Source: three-view drawing plus pictorial views. Frame: mm from the lowest corner of the part. A direction names the side the tool comes from. Give positions to 0.01 mm unless a question says otherwise; leave off trailing zeros. Loops run counter-clockwise (first coordinate to the right, second up) from the corner with the lowest first, then second, coordinate; pieces in that order, holes last. Notation, with made-up numbers: (80, 34) - (105, 34) arc R24 cw to (105, 49) - close; hole circle Ø1 at (7.5, 84.25). An arc over 180 degrees is marked (long way). Answer as a JSON object with one key per item and string values.
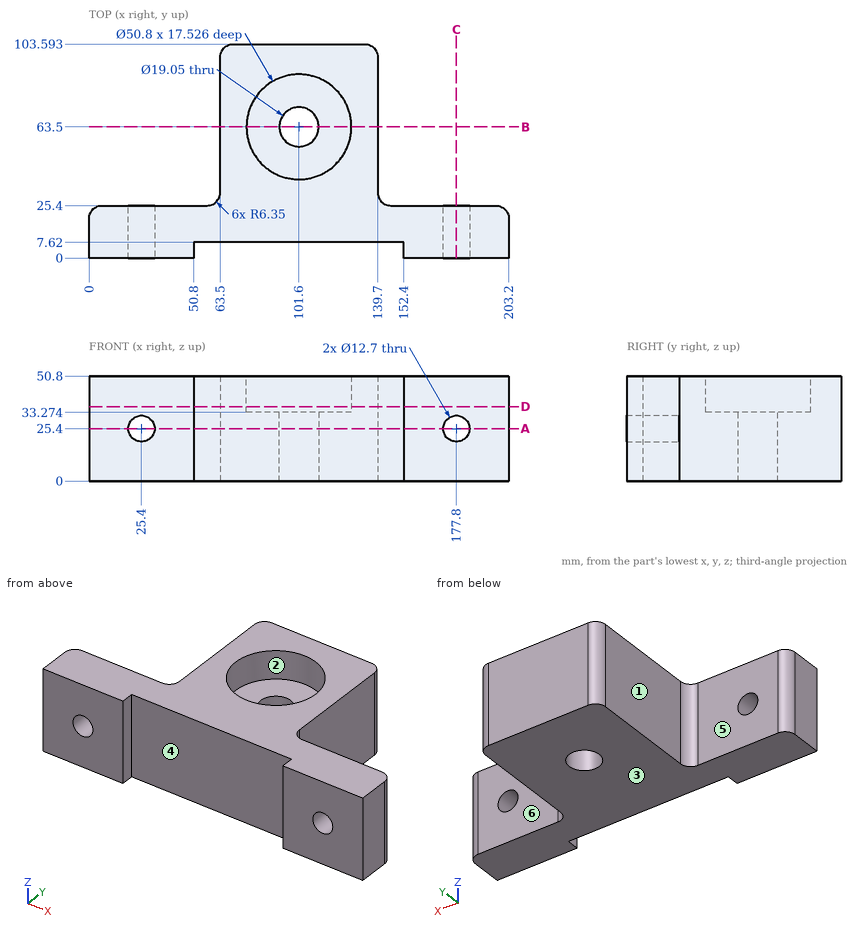
Item 1: Cut plane C-C (x = 177.8). Return loops of the section in (y, z).
Geometry check:
{"outline": "(0, 0) - (25.4, 0) - (25.4, 19.05) - (0, 19.05) - close; (0, 31.75) - (25.4, 31.75) - (25.4, 50.8) - (0, 50.8) - close"}
Item 2: Contact query for flat-ended pins moving along their axis: P1, Ø15, axis at x = 104, y = 63.5, coming from the +Z side; P2, Ø1, axis at y = 48, z = 6.5, coming from the +X side; P3, Ø15, axis at x = 25.5, z = 15, coming from the +Y side; P4, Ø10, axis at x = 177.8, z = 25.4, coming from the +Y side (1 decimal). Output: stop coordinate, or through.
Geometry check:
{"P1": "stops at z = 33.27", "P2": "stops at x = 139.7", "P3": "stops at y = 25.4", "P4": "passes through"}
Item 3: Material intervals for line 1 (X direction, y = 9, z = 25); line 2 (X direction, y = 63, z = 26); line 3 (Y direction, x = 101.6, z = 13) (1 decimal), sorted ascending. Write a range as [from, to].
Geometry check:
{"line 1": "x = [0, 19.06], [31.74, 171.46], [184.14, 203.2]", "line 2": "x = [63.5, 92.09], [111.11, 139.7]", "line 3": "y = [7.6, 54], [73, 103.6]"}
Item 4: Cut plane A-A (z = 25.4). Give the number of separate pieces and of enclosed holes in the cut face, then the cut area to 3 significant figures.
Geometry check:
{"separate pieces": "3", "enclosed holes": "1", "area": "9,400 mm2"}
Item 5: Mould query, pull axis X, two halves, no side actions, for the marked faces 1, 2 and 3. Classes: released by +X, released by -X, zero draft, split by the parting line, or undercut.
Geometry check:
{"face 1": "released by -X", "face 2": "undercut", "face 3": "zero draft"}
Item 6: Cut plane D-D (z = 36). Return loops of the section in (x, y), then the cut area to 3 significant figures.
Geometry check:
{"outline": "(0, 0) - (50.8, 0) - (50.8, 7.62) - (152.4, 7.62) - (152.4, 0) - (203.2, 0) - (203.2, 19.05) arc R6.35 ccw to (196.85, 25.4) - (146.05, 25.4) arc R6.35 cw to (139.7, 31.75) - (139.7, 97.24) arc R6.35 ccw to (133.35, 103.59) - (69.85, 103.59) arc R6.35 ccw to (63.5, 97.24) - (63.5, 31.75) arc R6.35 cw to (57.15, 25.4) - (6.35, 25.4) arc R6.35 ccw to (0, 19.05) - close; hole circle Ø50.8 at (101.6, 63.5)", "area": "8,300 mm2"}
Item 7: Cut plane B-B (y = 63.5). Return loops of the section in (x, z) (1 decimal), then the cut area to 3 significant figures.
Geometry check:
{"outline": "(63.5, 0) - (92.1, 0) - (92.1, 33.3) - (76.2, 33.3) - (76.2, 50.8) - (63.5, 50.8) - close; (111.1, 0) - (139.7, 0) - (139.7, 50.8) - (127, 50.8) - (127, 33.3) - (111.1, 33.3) - close", "area": "2,350 mm2"}
Item 8: Access query for the marked faces 4, 5 and 6. Directions: +Z, -Z, +X, -X, +Y, -Y. A direction counts if a zero-diameter tool reaches every point of the face in a straight line with its end or side. Return the directions, or none.
Geometry check:
{"face 4": "+Z, -Z, -Y", "face 5": "+Z, -Z, -X, +Y", "face 6": "+Z, -Z, +X, +Y"}
